Verification items for the finished model (mm, model axes). Round coordinates to 2 decimals unless told otherwise and drop trailing zeros. Write each loop counter-clockwise with the first axis right and the second up, starting at its lowest first coordinate (ties: lowest second). Pieces come first, ordered by that corner, then holes. Notation, with made-up numbers: (61, 30) - (86, 30) arc R34 ccw to (86, 60) - close; hole circle Ø7 at (40, 73). An arc over 180 degrees is marked (long way). Answer as a JSON object with one key per item and string values.
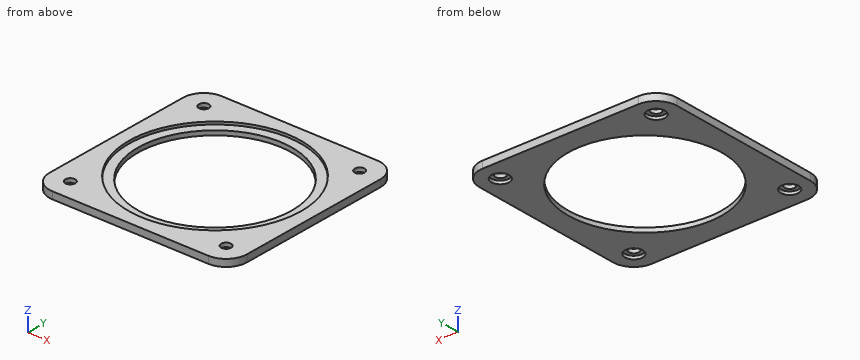
```python
from build123d import *

# Parameters (mm, degrees)
SKETCH1_R           = 73.75
SKETCH1_R_2         = 4.7625
BOSS_EXTRUDE1_DEPTH = 6.75
SKETCH2_R           = 8.5
CUT_EXTRUDE1_DEPTH  = 3
SKETCH3_R           = 82.55
CUT_EXTRUDE2_DEPTH  = 2.5


with BuildPart() as part:
    # Sketch1 → Boss-Extrude1 (new body)
    with BuildSketch(Plane.XY):
        with BuildLine():
            Line((75, -95), (-75, -95))
            ThreePointArc((-75, -95), (-89.142135624, -89.142135624), (-95, -75))
            Line((-95, -75), (-95, 75))
            ThreePointArc((-95, 75), (-89.142135624, 89.142135624), (-75, 95))
            Line((-75, 95), (75, 95))
            ThreePointArc((75, 95), (89.142135624, 89.142135624), (95, 75))
            Line((95, 75), (95, -75))
            ThreePointArc((95, -75), (89.142135624, -89.142135624), (75, -95))
        make_face()
        Circle(SKETCH1_R, mode=Mode.SUBTRACT)
        with Locations((-75, 75)):
            Circle(SKETCH1_R_2, mode=Mode.SUBTRACT)
        with Locations((75, 75)):
            Circle(SKETCH1_R_2, mode=Mode.SUBTRACT)
        with Locations((75, -75)):
            Circle(SKETCH1_R_2, mode=Mode.SUBTRACT)
        with Locations((-75, -75)):
            Circle(SKETCH1_R_2, mode=Mode.SUBTRACT)
    extrude(amount=BOSS_EXTRUDE1_DEPTH)

    # Sketch2 → Cut-Extrude1 (cut)
    with BuildSketch(Plane(origin=(0, 0, 0), x_dir=(-1, 0, 0), z_dir=(0, 0, -1))):
        with Locations((-75, 75)):
            Circle(SKETCH2_R)
        with Locations((75, 75)):
            Circle(SKETCH2_R)
        with Locations((75, -75)):
            Circle(SKETCH2_R)
        with Locations((-75, -75)):
            Circle(SKETCH2_R)
    extrude(amount=-CUT_EXTRUDE1_DEPTH, mode=Mode.SUBTRACT)

    # Sketch3 → Cut-Extrude2 (cut)
    with BuildSketch(Plane.XY.offset(6.75)):
        Circle(SKETCH3_R)
    extrude(amount=-CUT_EXTRUDE2_DEPTH, mode=Mode.SUBTRACT)


solid = part.part
```
Q1. Gauge pin test, flat end, axial feed: P1, Ø8.5, axis at x = -74.5, y = -76, coming from the -Z side. Record the tip position at first contact, or that the pin passes through.
Geometry check:
{"P1": "stops at z = 3"}
Q2. Section check C-C, the plane z = 1.75. Record the cut outline in (x, y), then the cut area to 3 significant figures.
Geometry check:
{"outline": "(-95, -75) arc R20 ccw to (-75, -95) - (75, -95) arc R20 ccw to (95, -75) - (95, 75) arc R20 ccw to (75, 95) - (-75, 95) arc R20 ccw to (-95, 75) - close; hole circle Ø17 at (-75, -75); hole circle Ø17 at (-75, 75); hole circle Ø147.5 at (0, 0); hole circle Ø17 at (75, -75); hole circle Ø17 at (75, 75)", "area": "17,800 mm2"}
Q3. Material ranges on line 1 along Y through (x, z) = (75, 4.55); line 2 along X through (y, z) = (0, 2.5), recorded low to high. Write a range as [from, to].
Geometry check:
{"line 1": "y = [-95, -79.76], [-70.24, -34.49], [34.49, 70.24], [79.76, 95]", "line 2": "x = [-95, -73.75], [73.75, 95]"}
Q4. Section check A-A, the plane x = 0. Record the cut outline in (y, z).
Geometry check:
{"outline": "(-95, 0) - (-73.75, 0) - (-73.75, 4.25) - (-82.55, 4.25) - (-82.55, 6.75) - (-95, 6.75) - close; (73.75, 0) - (95, 0) - (95, 6.75) - (82.55, 6.75) - (82.55, 4.25) - (73.75, 4.25) - close"}
